Here's how the part is built. I have some questions about the finished solid (model axes, mm). A direction names the side the tool comes from. Coordinates: 2 decimals unless noted, no trailing zeros. Write each loop counter-clockwise with the first axis right and the second up, starting at its lowest first coordinate (ties: lowest second). Pieces come first, ordered by that corner, then holes. Notation, with made-up numbers: (24, -11) - (32, -11) arc R14 cw to (32, 7) - close; hole circle Ø8 at (-21, 58.5). An arc over 180 degrees is marked (long way). Answer in a Markdown table with one row per item. Add a question column.
Item 1: Imagine slicing it at D-D (z = -64). State how many separate pieces and enclosed holes the cut face has, plus the area to 3 significant figures.
Item 2: We'd pull the mould along Z, two halves only. Please class faces 1 (the face through (25.4, 309, -13)), 2 (the face through (13, 301, -25.4)), 3 (the face through (607.185, 430.253, 32.017)): +Z half, -Z half, draft (parallel to the pull), parting line (faces both ways), or undercut.
Item 3: Which directions (+Z, -Z, +X, -X, +Y, -Y) give clear straight access to the entire face, cutting with the end or side of a thin tool? Please do faces 4 (the face through (4.762, 301, 12)), 5 (the face through (25.4, 13, -389)), 6 (the face through (25.4, 309, -775)), 7 (the face through (2.348, 430.253, 32.017)), 8 (the face through (13, 584.2, -389)).
Item 4: I'm going to push flat-ended pins straight in: pin 1 (1 mm diameter, centred on x = 96, y = 141.5, fed in from +Z); pin 2 (12.5 mm diameter, centred on y = 165.5, z = -780, fed in from -X); pin 3 (2 mm diameter, centred on x = 548, y = 181.5, fed in from -Z). Where does each tip first touch, or does it pass through?
Item 5: Imagine slicing it at B-B (x = 128). Please give me the cut outline in (y, z).
Item 6: Imagine slicing it at A-A (z = -196). Please give me the cut outline in (x, y).
Item 7: If I drill on probe 1 along Z at (x, y) = (564, 146); probe 2 along Z at (x, y) = (316, 257); probe 3 along X at (y, z) = (414, -67) (3 decimals), over which ranges is the centre line in solid material (lowest first)? Write a range as from..to.
from build123d import *

# Parameters (mm, degrees)
F0_W      = 609.6
F0_H      = 609.6
F1_DEPTH  = 50.8
F2_W      = 304.8
F2_H      = 304.8
F4_W      = 228.6
F4_H      = 228.6
F6_T      = -4.7625
F7_W      = 609.6
F7_H      = 609.6
F7_W_2    = 558.8
F7_H_2    = 558.8
F8_DEPTH  = 25.4
F10_DEPTH = 609.601
F11_W     = 25.4
F11_H     = 25.4
F12_DEPTH = 762
F13_W     = 609.6
F13_H     = 609.6
F13_W_2   = 558.8
F13_H_2   = 558.8
F14_DEPTH = 25.4


with BuildPart() as f1:
    # F0 (on Top) → F1 (new body)
    with BuildSketch(Plane.XY):
        with Locations((304.8, 304.8)):
            Rectangle(F0_W, F0_H)
    extrude(amount=F1_DEPTH)

    # F2 (on face) → F5 section 0
    with BuildSketch(Plane(origin=(0, 0, 0), x_dir=(1, 0, 0), z_dir=(0, 0, -1))):
        with Locations((304.8, -304.8)):
            Rectangle(F2_W, F2_H)
    # F4 (on offset) → F5 section 1
    with BuildSketch(Plane(origin=(0, 0, -101.6), x_dir=(1, 0, 0), z_dir=(0, 0, -1))):
        with Locations((304.8, -304.8)):
            Rectangle(F4_W, F4_H)
    loft()

    # F6
    f6_openings = [f1.faces().sort_by_distance(p)[0] for p in [
        (304.8, 304.8, 50.8),
    ]]
    offset(amount=F6_T, openings=f6_openings, kind=Kind.INTERSECTION)

    # F7 (on face) → F8 (join)
    with BuildSketch(Plane(origin=(0, 0, 0), x_dir=(1, 0, 0), z_dir=(0, 0, -1))):
        with Locations((304.8, -304.8)):
            Rectangle(F7_W, F7_H)
        with Locations((304.8, -304.8)):
            Rectangle(F7_W_2, F7_H_2, mode=Mode.SUBTRACT)
    extrude(amount=F8_DEPTH)

    # F9 (on face) → F10 (cut, through all)
    with BuildSketch(Plane(origin=(0, 0, 0), x_dir=(0, -1, 0), z_dir=(-1, 0, 0))):
        Polygon((-441.0970452561, 50.8), (-419.1, 12.7), (-190.5, 12.7), (-168.5029547439, 50.8), align=None)
    extrude(amount=-F10_DEPTH, mode=Mode.SUBTRACT)

    # F11 (on face) → F12 (join)
    with BuildSketch(Plane(origin=(0, 0, -25.4), x_dir=(1, 0, 0), z_dir=(0, 0, -1))):
        with Locations((12.7, -12.7)):
            Rectangle(F11_W, F11_H)
        with Locations((596.9, -12.7)):
            Rectangle(F11_W, F11_H)
        with Locations((596.9, -596.9)):
            Rectangle(F11_W, F11_H)
        with Locations((12.7, -596.9)):
            Rectangle(F11_W, F11_H)
    extrude(amount=F12_DEPTH)

    # F13 (on face) → F14 (join)
    with BuildSketch(Plane(origin=(0, 0, -787.4), x_dir=(1, 0, 0), z_dir=(0, 0, -1))):
        with Locations((304.8, -304.8)):
            Rectangle(F13_W, F13_H)
        with Locations((304.8, -304.8)):
            Rectangle(F13_W_2, F13_H_2, mode=Mode.SUBTRACT)
    extrude(amount=-F14_DEPTH)


solid = f1.part
Here are the results:
| question | item | result |
|---|---|---|
| 1 | separate pieces | 5 |
| 1 | enclosed holes | 1 |
| 1 | area | 7,700 mm2 |
| 2 | face 1 | draft |
| 2 | face 2 | undercut |
| 2 | face 3 | +Z half |
| 3 | face 4 | +Z |
| 3 | face 5 | +Y, -Y |
| 3 | face 6 | -Z |
| 3 | face 7 | +Z, +X, -X |
| 3 | face 8 | +X, -X |
| 4 | pin 1 | stops at z = 4.76 |
| 4 | pin 2 | stops at x = 0 |
| 4 | pin 3 | stops at z = 0 |
| 5 | outline | (0, -787.4) - (25.4, -787.4) - (25.4, -762) - (0, -762) - close; (0, -25.4) - (25.4, -25.4) - (25.4, 0) - (584.2, 0) - (584.2, -25.4) - (609.6, -25.4) - (609.6, 50.8) - (604.84, 50.8) - (604.84, 4.76) - (4.76, 4.76) - (4.76, 50.8) - (0, 50.8) - close; (584.2, -787.4) - (609.6, -787.4) - (609.6, -762) - (584.2, -762) - close |
| 6 | outline | (0, 0) - (25.4, 0) - (25.4, 25.4) - (0, 25.4) - close; (0, 584.2) - (25.4, 584.2) - (25.4, 609.6) - (0, 609.6) - close; (584.2, 0) - (609.6, 0) - (609.6, 25.4) - (584.2, 25.4) - close; (584.2, 584.2) - (609.6, 584.2) - (609.6, 609.6) - (584.2, 609.6) - close |
| 7 | probe 1 | z = 0..4.76 |
| 7 | probe 2 | z = -101.6..-96.84 |
| 7 | probe 3 | x = 177.525..182.611, 426.989..432.075 |
